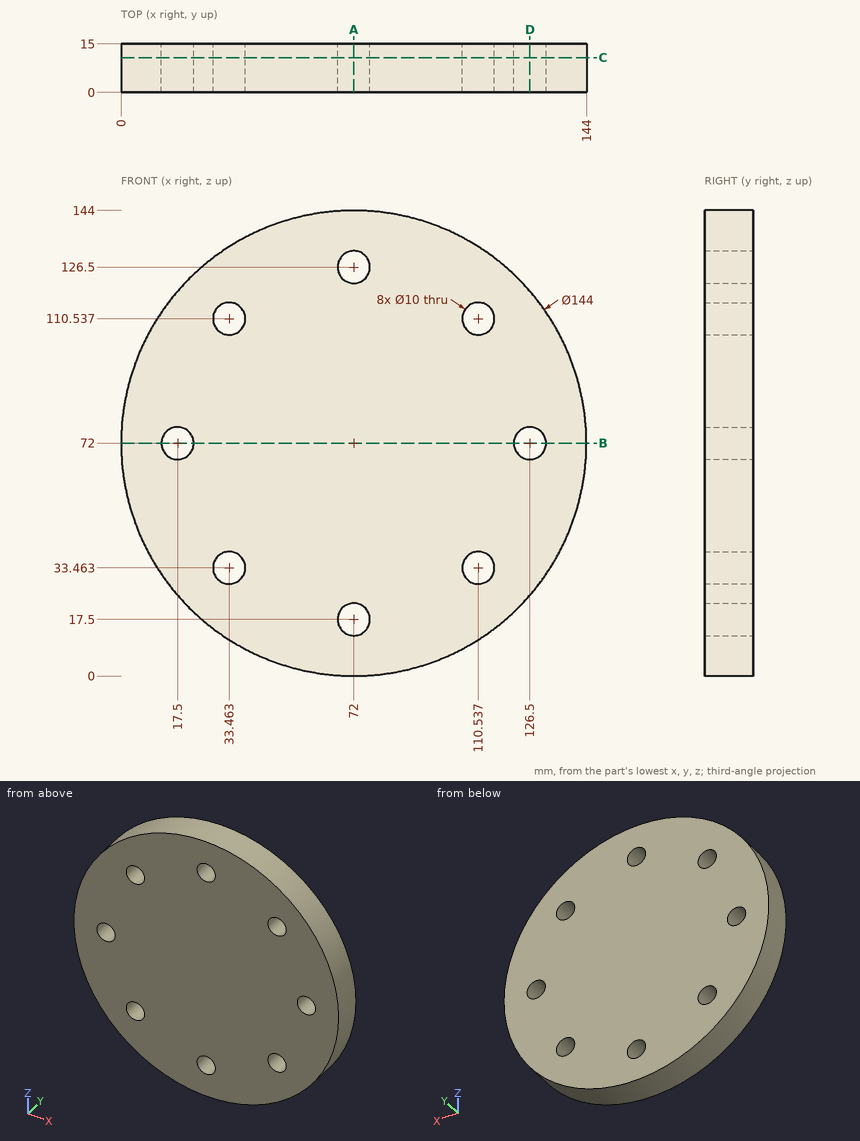
Check sheet for the drawn part. Datum: minimum x, y, z corner. Units: mm. Round coordinates to 2 decimals unless told otherwise and drop trailing zeros. Write each loop counter-clockwise with the first axis right and the second up, starting at its lowest first coordinate (ties: lowest second). Pieces come first, ordered by that corner, then holes. Notation, with made-up numbers: (24, 83.25) - (52, 83.25) arc R26 cw to (52, 97.25) - close; hole circle Ø1 at (76, -35). An arc over 180 degrees is marked (long way). Return JSON: item names as keys, results as strings.
Q1. Scan lines: L1, parallel to Z at x = 72, y = 5.75; L2, parallel to X at y = 14, z = 68.5 (1 decimal). Record each from-to range of solid material in increasing order. Write a range as from..to.
Returned:
{"L1": "z = 0..12.5, 22.5..121.5, 131.5..144", "L2": "x = 0.1..13.9, 21.1..122.9, 130.1..143.9"}
Q2. Cross-section at A-A (x = 72). Record the boundary of the cut face in (y, z), then the cut area to 3 significant figures.
Returned:
{"outline": "(0, 0) - (15, 0) - (15, 12.5) - (0, 12.5) - close; (0, 22.5) - (15, 22.5) - (15, 121.5) - (0, 121.5) - close; (0, 131.5) - (15, 131.5) - (15, 144) - (0, 144) - close", "area": "1,860 mm²"}
Q3. Cross-section at B-B (z = 72). Record the boundary of the cut face in (x, y), then the cut area to 3 significant figures.
Returned:
{"outline": "(0, 0) - (12.5, 0) - (12.5, 15) - (0, 15) - close; (22.5, 0) - (121.5, 0) - (121.5, 15) - (22.5, 15) - close; (131.5, 0) - (144, 0) - (144, 15) - (131.5, 15) - close", "area": "1,860 mm²"}
Q4. Cross-section at D-D (x = 126.5). Record the boundary of the cut face in (y, z), then the cut area to 3 significant figures.
Returned:
{"outline": "(0, 24.95) - (15, 24.95) - (15, 67) - (0, 67) - close; (0, 77) - (15, 77) - (15, 119.05) - (0, 119.05) - close", "area": "1,260 mm²"}
Q5. Depth check by flat-ended pin: P1, Ø8, axis at x = 110.54, z = 110.54, coming from the -Y side; P2, Ø11.5, axis at x = 72, z = 126.5, coming from the -Y side; P3, Ø6, axis at x = 68, y = 7, coming from the +Z side; P4, Ø1, axis at y = 8.5, z = 64, coming from the -X side. Enter the tip coordinate at first touch or a pass-through.
Returned:
{"P1": "passes through", "P2": "stops at y = 0", "P3": "stops at z = 143.99", "P4": "stops at x = 0.39"}
Q6. Cross-section at C-C (y = 10.75). Give the number of separate pieces and of enclosed holes in the cut face, then the cut area to 3 significant figures.
Returned:
{"separate pieces": "1", "enclosed holes": "8", "area": "15,700 mm²"}
